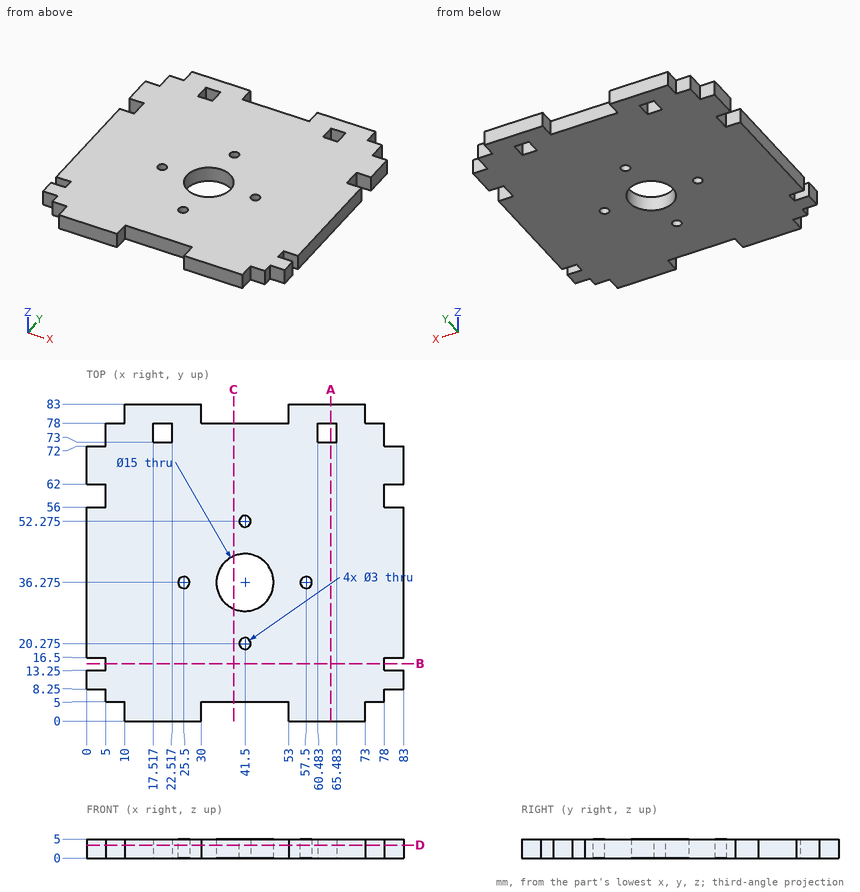
Verification items for this drawing (mm, ordinates from the low corner). Coordinates: 2 decimals unless noted, no trailing zeros. Loops run counter-clockwise (first coordinate to the right, second up) from the corner with the lowest first, then second, coordinate; pieces in that order, holes last. Notation, with made-up numbers: (-28, 19.25) - (-24, 19.25) arc R29 ccw to (-24, 45.25) - close; hole circle Ø2 at (45.25, 77.5). An arc over 180 degrees is marked (long way). Use one line per item in the form item = value. Start each with the question number.
Item 1: Thickness scan on probe 1 along X at (y, z) = (74.5, 1.4); probe 2 along Y at (x, z) = (41.5, 2.25) (1 decimal); probe 3 along Y at (x, z) = (42.5, 3.65). Record the ranges inside material, lowest first.
Item 2: Section check D-D, the plane z = 3.4. Give the number of separate pieces and of enclosed holes in the cut face, and give its area (3 significant figures).
Item 3: Section check C-C, the plane x = 38.5. Enter the section's corners in (y, z), and give its area (3 significant figures).
Item 4: Section check A-A, the plane x = 64. Enter the section's corners in (y, z), and give its area (3 significant figures).
Item 5: Section check B-B, the plane y = 15. Enter the section's corners in (x, z).
Item 6: Gauge pin test, flat ends, axial feed: pin 1 (1.5 mm diameter, centred on y = 80, z = 1.5, fed in from -X); pin 2 (2 mm diameter, centred on y = 14, z = 3, fed in from +X); pin 3 (1.6 mm diameter, centred on y = 14.5, z = 3, fed in from +X); pin 4 (1.5 mm diameter, centred on x = 81.5, z = 2.5, fed in from +Y). Record the tip position at first contact, or that the pin passes through.
Computed:
q1.probe_1 = 5 to 17.52, 22.52 to 60.48, 65.48 to 78
q1.probe_2 = 5 to 18.8, 21.8 to 28.8, 43.8 to 50.8, 53.8 to 78
q1.probe_3 = 5 to 19.16, 21.39 to 28.84, 43.71 to 51.16, 53.39 to 78
q2.separate_pieces = 1
q2.enclosed_holes = 7
q2.area = 6,020 mm2
q3.outline = (5, 0) - (29.4, 0) - (29.4, 5) - (5, 5) - close; (43.15, 0) - (78, 0) - (78, 5) - (43.15, 5) - close
q3.area = 296 mm2
q4.outline = (0, 0) - (73, 0) - (73, 5) - (0, 5) - close; (78, 0) - (83, 0) - (83, 5) - (78, 5) - close
q4.area = 390 mm2
q5.outline = (5, 0) - (78, 0) - (78, 5) - (5, 5) - close
q6.pin_1 = 10
q6.pin_2 = 83
q6.pin_3 = 78
q6.pin_4 = 72
